```python
from build123d import *

# Parameters (mm, degrees)
SALIENTE_EXTRUIR1_DEPTH    = 30
CORTAR_EXTRUIR1_DEPTH      = 25
CROQUIS4_W                 = 24.5
CROQUIS4_H                 = 24.5
SALIENTE_EXTRUIR2_DEPTH    = 5
CROQUIS5_W                 = 40
CROQUIS5_H                 = 40
CROQUIS5_W_2               = 20
SALIENTE_EXTRUIR4_DEPTH    = 40
CORTAR_EXTRUIR5_DEPTH      = 59.309518948
CORTAR_EXTRUIR5_DEPTH_BACK = 59.309518948
CROQUIS9_R                 = 5


with BuildPart() as part:
    # Croquis1 → Saliente-Extruir1 (new body)
    with BuildSketch(Plane.XY):
        Polygon((-5, 5), (35, 5), (35, -10.5), (10.5, -10.5), (10.5, -35), (-5, -35), align=None)
    extrude(amount=SALIENTE_EXTRUIR1_DEPTH)

    # Croquis3 → Cortar-Extruir1 (cut)
    with BuildSketch(Plane.XY.offset(30)):
        Polygon((0, -30), (0, -35), (5.5, -35), (5.5, -30), (5.5, -5.5), (30, -5.5), (35, -5.5), (35, 0), (30, 0), (0, 0), align=None)
    extrude(amount=-CORTAR_EXTRUIR1_DEPTH, mode=Mode.SUBTRACT)

    # Croquis4 → Saliente-Extruir2 (add)
    with BuildSketch(Plane(origin=(0, 0, 0), x_dir=(-1, 0, 0), z_dir=(0, 0, -1))):
        with Locations((-22.75, -22.75)):
            Rectangle(CROQUIS4_W, CROQUIS4_H)
    extrude(amount=-SALIENTE_EXTRUIR2_DEPTH)

    # Croquis5 → Saliente-Extruir4 (add)
    with BuildSketch(Plane(origin=(0, 0, 0), x_dir=(-1, 0, 0), z_dir=(0, 0, -1))):
        with Locations((-15, -15)):
            Rectangle(CROQUIS5_W, CROQUIS5_H)
        with Locations((-45, -15)):
            Rectangle(CROQUIS5_W_2, CROQUIS5_H)
        Polygon((5, -55), (5, -35), (-35, -35), (-55, -35), (-55, -55), align=None)
    extrude(amount=SALIENTE_EXTRUIR4_DEPTH)

    # Croquis9 → Cortar-Extruir5 (cut, two sides: drawn at the far end of the back side and taken through both)
    with BuildSketch(Plane(origin=(25, -25, 0), x_dir=(0, 0, 1), z_dir=(0.7071067811865487, -0.7071067811865465, 0)).offset(-CORTAR_EXTRUIR5_DEPTH_BACK)):
        with Locations(Location((-20, 0, 0), (0, 0, 180))):
            Circle(CROQUIS9_R)
    extrude(amount=CORTAR_EXTRUIR5_DEPTH + CORTAR_EXTRUIR5_DEPTH_BACK, mode=Mode.SUBTRACT)


solid = part.part
```
Can you work these out from the model? Positions are in its coordinate system, mm. A direction names the side the tool comes from. Give positions to 0.01 mm unless a question says otherwise; leave off trailing zeros. Order: outer loops, then holes, each group sorted by start corner. A loop starts at its lowest first (then second) coordinate and runs counter-clockwise, first axis right, second up. Notation, with made-up numbers: M -7.5,-9 L 28.5,-9 A17 ccw 28.5,1 Z; hole C -9,-14 d10. An arc over 180 degrees is marked long. Write item = value, one per line. Start each with the question number.
Q1. We'd pull the mould along X, two halves only. Please class faces 4 (the flat face through (25, -25, -40)), 5 (the flat face through (-5, -25, -5)), 6 (the flat face through (10, -4, 5)): pulls with the +X half, pulls with the -X half, needs draft (parallel to the pull), parting line crosses it, or undercut.
Q2. For faces 1 (the flat face through (0, -17, 18)), 2 (the flat face through (23, -23, 5)), 3 (the flat face through (6, -35, 8)), which set-ups out of +Z, -Z, +X, -X, +Y, -Y let a thin tool reach every point of the face, with its end or its side?
Q3. Suppose I cut it at C-C (z = -17). Write out the boundary of the cut face in (x, y).
Q4. Will these pins go through, and if not, where does the flat tip stop? pin 1 Ø17.5 at (x, y) = (26, -25.5) entering from +Z; pin 2 Ø12.5 at (x, z) = (20.5, 19) entering from -Y; pin 3 Ø20 at (y, z) = (-20, 14) entering from +X.
Q5. Suppose I cut it at B-B (z = 4). Write out the boundary of the cut face in (x, y).
Q6. I need wall thicknesses on probe 1 along Y at (x, z) = (14.5, 11.5); probe 2 along X at (y, z) = (-20, 6.5); probe 3 along Y at (x, z) = (8, 23.5). Which ranges of each line are inside material? Lowest first, please. Write a range as [from, to].
Q7. Suppose I cut it at A-A (z = 12). Write out the boundary of the cut face in (x, y).
Check result:
q1.face_4 = needs draft
q1.face_5 = pulls with the -X half
q1.face_6 = undercut
q2.face_1 = +Z, -Y
q2.face_2 = +Z, +X, -Y
q2.face_3 = +Z, +X, -X, -Y
q3.outline = M -5,-55 L 49.34,-55 L -5,-0.66 Z; M 0.66,5 L 55,-49.34 L 55,5 Z
q4.pin_1 = 5
q4.pin_2 = -10.5
q4.pin_3 = 35
q5.outline = M -5,-35 L 35,-35 L 35,5 L -5,5 Z
q6.probe_1 = [-10.5, -5.5], [0, 5]
q6.probe_2 = [-5, 0], [5.5, 10.5]
q6.probe_3 = [-35, -5.5], [0, 5]
q7.outline = M -5,-35 L 0,-35 L 0,0 L 35,0 L 35,5 L -5,5 Z; M 5.5,-35 L 10.5,-35 L 10.5,-10.5 L 35,-10.5 L 35,-5.5 L 5.5,-5.5 Z
